Autodesk Inventor part; units mm, degrees
ref_plane "YZ Plane" through (0, 0, 0) normal (1, 0, 0) x (0, 1, 0)
ref_plane "XZ Plane" through (0, 0, 0) normal (0, 1, 0) x (-1, 0, 0)
ref_plane "XY Plane" through (0, 0, 0) normal (0, 0, 1) x (1, 0, 0)
sketch "스케치1" plane through (0, 0, 0) normal (0, 1, 0) x (-1, 0, 0)
  line L0 (60, 80) -> (-60, 80)
  line L1 (-60, 80) -> (-60, -80)
  line L2 (-60, -80) -> (60, -80)
  line L3 (60, -80) -> (60, 80)
  line L4 (60, 80) -> (-60, -80) construction
  line L5 (-60, 80) -> (60, -80) construction
  point P0 (0, 0)
  dimension "d0" = 120
  dimension "d1" = 160
extrude "돌출1" add sketch "스케치1" along normal blind 60
sketch "스케치2" plane through (0, 60, 0) normal (0, 1, 0) x (1, 0, 0)
  line L0 (60, -80) -> (60, 80)
  line L1 (60, 80) -> (-60, 80)
  line L2 (55, 102.1646) -> (-55, 102.1646)
  line L3 (-55, 102.1646) -> (-55, -89.711)
  line L4 (-55, -89.711) -> (55, -89.711)
  line L5 (55, -89.711) -> (55, 102.1646)
  line L6 (-60, 80) -> (-60, -80)
  point P0 (0, 0)
  point P1 (55, 80)
  point P2 (-55, 80)
  dimension "d6" = 5
  dimension "d7" = 5
extrude "돌출2" cut sketch "스케치2" against normal blind 40 contours L5 L4 L3 L1
sketch "스케치12" plane through (60, 0, -80) normal (0, 0, -1) x (-1, 0, 0)
  line L0 (-34.8463, 10) -> (156.2634, 10)
  line L1 (156.2634, 10) -> (156.2634, -36.9465)
  line L2 (156.2634, -36.9465) -> (-34.8463, -36.9465)
  line L3 (-34.8463, -36.9465) -> (-34.8463, 10)
  line L4 (0, 0) -> (120, 0)
  point P0 (60, 0)
  dimension "d85" = 10
extrude "돌출10" cut sketch "스케치12" against normal through all
sketch "스케치13" plane through (-55, 20, 80) normal (0, 0, 1) x (1, 0, 0)
  line L0 (0, 40) -> (0, 0)
  line L1 (0, 0) -> (110, 0)
  line L2 (0, 40) -> (110, 40)
  line L3 (110, 40) -> (110, 0)
  line L4 (110, 0) -> (0, 0)
  line L5 (0, 0) -> (0, 40)
  point P0 (55, -20)
extrude "돌출11" add sketch "스케치13" against normal blind 5
sketch "스케치14" plane through (55, 20, -80) normal (0, 0, -1) x (-1, 0, 0)
  line L0 (0, 0) -> (0, 40)
  line L1 (110, 0) -> (0, 0)
  line L2 (0, 40) -> (110, 40)
  line L3 (110, 40) -> (110, 0)
  line L4 (110, 0) -> (0, 0)
  line L5 (0, 0) -> (0, 40)
  point P0 (55, -20)
extrude "돌출12" add sketch "스케치14" against normal blind 5
sketch "스케치15" plane through (60, 60, -80) normal (0, 0, -1) x (-1, 0, 0)
  point P0 (60, -60)
sketch "스케치16" plane through (60, 60, -80) normal (0, 0, -1) x (-1, 0, 0)
  point P0 (60, -60)
sketch "스케치17" plane through (0, 20, 0) normal (0, 1, 0) x (1, 0, 0)
  line L0 (7, 27) -> (45, 27)
  line L1 (45, 27) -> (45, 65)
  line L2 (45, 65) -> (7, 65)
  line L3 (7, 65) -> (7, 27)
  line L4 (55, 75) -> (55, -75)
  line L5 (55, 75) -> (-55, 75)
  circle A0 centre (7, 27) radius 1.6
  circle A1 centre (7, 65) radius 1.6
  circle A2 centre (45, 65) radius 1.6
  circle A3 centre (45, 27) radius 1.6
  line L6 (-47.9371, 14.7215) -> (-7.9371, 14.7215)
  line L7 (-7.9371, 14.7215) -> (-7.9371, 64.7215)
  line L8 (-7.9371, 64.7215) -> (-47.9371, 64.7215)
  line L9 (-47.9371, 64.7215) -> (-47.9371, 14.7215)
  point P0 (0, 0)
  dimension "d92" = 38
  dimension "d93" = 38
  dimension "d95" = 10
  dimension "d96" = 10
  dimension "d97" = 3.2
  dimension "d98" = 3.2
  dimension "d99" = 3.2
  dimension "d100" = 3.2
  dimension "d113" = 40
  dimension "d114" = 50
extrude "돌출13" cut sketch "스케치17" against normal through all contours L3 A0 L0 | L0 A0 L3 | A3 L1 L0 | L0 L1 A3 | A1 L2 L3 | L3 L2 A1 | A2 L2 L1 | L1 L2 A2
sketch "스케치19" plane through (60, 60, -80) normal (0, 0, -1) x (-1, 0, 0)
  line L0 (5, -40) -> (115, -40)
  circle A0 centre (46.5, -25) radius 8.5
  circle A1 centre (73.5, -25) radius 8.5
  line L1 (5, 0) -> (5, -40)
  line L2 (115, -40) -> (115, 0)
  point P0 (60, -60)
  dimension "d105" = 27
  dimension "d106" = 41.5
  dimension "d107" = 17
  dimension "d108" = 17
  dimension "d109" = 15
  dimension "d110" = 15
extrude "돌출14" cut sketch "스케치19" against normal through all
sketch "스케치21" plane through (0, 20, 0) normal (0, 1, 0) x (1, 0, 0)
  circle A0 centre (5.4243, 8.1678) radius 7.5
  line L0 (-49.3888, 17.2731) -> (-9.3888, 17.2731)
  line L1 (-9.3888, 17.2731) -> (-9.3888, 67.2731)
  line L2 (-9.3888, 67.2731) -> (-49.3888, 67.2731)
  line L3 (-49.3888, 67.2731) -> (-49.3888, 17.2731)
  point P0 (0, 0)
  dimension "d117" = 15
  dimension "d118" = 50
  dimension "d119" = 40
extrude "돌출15" cut sketch "스케치21" against normal through all contours A0
sketch "스케치23" plane through (0, 20, 0) normal (0, 1, 0) x (1, 0, 0)
  line L0 (-48.6, -65) -> (20, -65)
  line L1 (20, -65) -> (20, -11.6)
  line L2 (20, -11.6) -> (-48.6, -11.6)
  line L3 (-48.6, -11.6) -> (-48.6, -65)
  line L4 (55, 75) -> (55, -75)
  line L5 (-55, -75) -> (55, -75)
  circle A0 centre (4.7, -62.45) radius 1.6
  circle A1 centre (6.03, -14.15) radius 1.6
  circle A2 centre (-46.05, -47.16) radius 1.6
  circle A3 centre (-46.05, -19.23) radius 1.6
  point P0 (0, 0)
  dimension "d123" = 68.6
  dimension "d124" = 53.4
  dimension "d125" = 35
  dimension "d126" = 10
  dimension "d127" = 3.2
  dimension "d128" = 15.3
  dimension "d129" = 2.55
  dimension "d130" = 3.2
  dimension "d131" = 13.97
  dimension "d132" = 2.55
  dimension "d133" = 3.2
  dimension "d134" = 35.56
  dimension "d135" = 3.2
  dimension "d136" = 2.55
  dimension "d137" = 2.55
  dimension "d138" = 7.63
extrude "돌출16" cut sketch "스케치23" against normal through all contours A0 | A1 | A2 | A3
sketch "스케치24" plane through (0, 20, 0) normal (0, 1, 0) x (1, 0, 0)
  line L0 (-55, -75) -> (55, -75)
  line L1 (55, 75) -> (55, -75)
  line L2 (-55, -75) -> (55, -75)
  line L3 (55, -75) -> (55, 75)
  line L4 (55, 75) -> (-55, 75)
  line L5 (-55, 75) -> (-55, -75)
  point P0 (0, 0)
extrude "돌출17" cut sketch "스케치24" against normal through all
properties part number "본체 겉면"
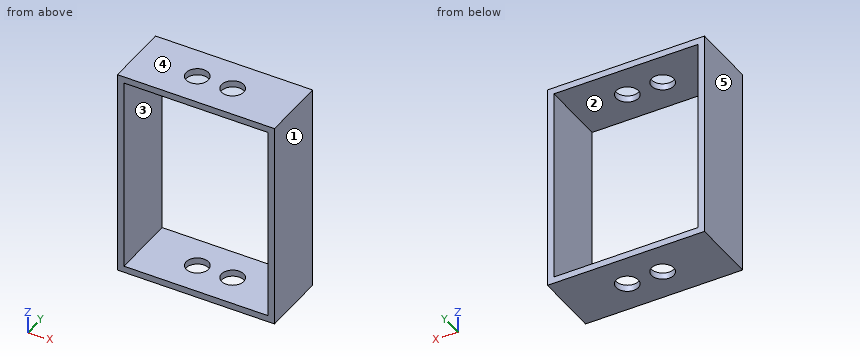
Build history of the part. All positions in model axes, mm. Face numbers are marked on the shaded views. A direction names the side the tool comes from. Give positions to 0.01 mm unless a question says otherwise; leave off trailing zeros. Loops run counter-clockwise (first coordinate to the right, second up) from the corner with the lowest first, then second, coordinate; pieces in that order, holes last. Notation, with made-up numbers: (36, -26) - (76, -26) arc R28 ccw to (76, 5) - close; hole circle Ø8 at (47, 2). An arc over 180 degrees is marked (long way). Write item = value, one per line. Start each with the question number.
1) Drop a flat-ended pin along its axis: pin 1 Ø10 at (x, y) = (-13.5, 35) entering from +Z. Give the stop position or say it passes through.
2) Band-saw the part on C-C on x = 13.5. Give the cut face in (y, z), plus the area to 3 significant figures.
3) Tool access for the marked faces 1 and 2: list every direction of +Z, -Z, +X, -X, +Y, -Y with a clear straight run to the whole face (end or side of a thin tool).
4) Pull direction Z, two halves, no side cores. Call the marked faces 3, 4 and 5: +Z half, -Z half, draft (parallel to the pull), parting line (faces both ways), or undercut.
5) Band-saw the part on A-A on y = 35. Give the cut face in (x, z).
6) Band-saw the part on B-B on z = -53.5. Give the cut face in (x, y).
7) Band-saw the part on D-D on x = -45.5. Give the cut face in (y, z).
8) Probe probe 1 along Z at (x, y) = (-17.5, 52); probe 2 along X at (y, z) = (21, 6.5); probe 3 along Y at (x, z) = (13.5, 77.85). List the from-to ranges inside material, lowest first. Write a range as from..to.
Final values:
q1.pin_1 = through
q2.outline = (10, -80) - (26.5, -80) - (26.5, -75) - (10, -75) - close; (10, 75) - (26.5, 75) - (26.5, 80) - (10, 80) - close; (43.5, -80) - (60, -80) - (60, -75) - (43.5, -75) - close; (43.5, 75) - (60, 75) - (60, 80) - (43.5, 80) - close
q2.area = 330 mm²
q3.face_1 = +Z, -Z, +X, +Y, -Y
q3.face_2 = +Y, -Y
q4.face_3 = undercut
q4.face_4 = +Z half
q4.face_5 = draft
q5.outline = (-60, -80) - (-22, -80) - (-22, -75) - (-55, -75) - (-55, 75) - (-22, 75) - (-22, 80) - (-60, 80) - close; (-5, -80) - (5, -80) - (5, -75) - (-5, -75) - close; (-5, 75) - (5, 75) - (5, 80) - (-5, 80) - close; (22, -80) - (60, -80) - (60, 80) - (22, 80) - (22, 75) - (55, 75) - (55, -75) - (22, -75) - close
q6.outline = (-60, 10) - (-55, 10) - (-55, 60) - (-60, 60) - close; (55, 10) - (60, 10) - (60, 60) - (55, 60) - close
q7.outline = (10, -80) - (60, -80) - (60, -75) - (10, -75) - close; (10, 75) - (60, 75) - (60, 80) - (10, 80) - close
q8.probe_1 = -80..-75, 75..80
q8.probe_2 = -60..-55, 55..60
q8.probe_3 = 10..26.5, 43.5..60
